```python
from build123d import *

# Parameters (mm, degrees)
SKETCH_1_R      = 1.6
EXTRUDE_1_DEPTH = 3
EXTRUDE_2_DEPTH = 10
SKETCH_3_R      = 1.6
EXTRUDE_3_DEPTH = 3


with BuildPart() as part:
    # 草图1 → 凸台-拉伸1 (new body)
    with BuildSketch(Plane(origin=(0, 0, 0), x_dir=(1, 0, 0), z_dir=(0, 1, 0))):
        with Locations(Location((0, 0, 0), (0, 0, 270))):
            Circle(SKETCH_1_R)
    extrude(amount=EXTRUDE_1_DEPTH)

    # 草图2 → 凸台-拉伸2 (add)
    with BuildSketch(Plane(origin=(0, 3, 0), x_dir=(1, 0, 0), z_dir=(0, 1, 0))):
        Polygon((2.757018897, -1.686460265), (2.839026881, 1.544418271), (0.082007983, 3.230878536), (-2.757018897, 1.686460265), (-2.839026881, -1.544418271), (-0.082007983, -3.230878536), align=None)
    extrude(amount=EXTRUDE_2_DEPTH)

    # 草图3 → 凸台-拉伸3 (add)
    with BuildSketch(Plane(origin=(0, 13, 0), x_dir=(1, 0, 0), z_dir=(0, 1, 0))):
        with Locations(Location((0, 0, 0), (0, 0, 270))):
            Circle(SKETCH_3_R)
    extrude(amount=EXTRUDE_3_DEPTH)


solid = part.part
```
Source: CAD feature listing. Evaluate the final solid. Frame: model axes, mm. A direction names the side the tool comes from. Give positions to 0.01 mm unless a question says otherwise; leave off trailing zeros. Loops run counter-clockwise (first coordinate to the right, second up) from the corner with the lowest first, then second, coordinate; pieces in that order, holes last. Notation, with made-up numbers: (46.25, -23.5) -> (66.25, -23.5) arc R9 cw to (66.25, -19.5) -> close; hole circle Ø11 at (52, -21.5). An arc over 180 degrees is marked (long way). Use a Markdown table: item, result. Add a question column.
(1) Access query for faces 1 (the face through (-0.97, 1.48, -1.27)), 2 (the face through (-1.48, 7.93, 2.376)), 3 (the face through (1.2, 13, 1.4)). Directions: +Z, -Z, +X, -X, +Y, -Y. A direction counts if a zero-diameter tool reaches every point of the face in a straight line with its end or side. Return the directions, or none.
(2) First-contact query: pin 1 Ø1 at (x, y) = (-2, 11) entering from +Z; pin 2 Ø1.5 at (x, y) = (1, 13) entering from +Z; pin 3 Ø1 at (y, z) = (12.5, 0) entering from -X. Flat tips, straight axial feed; report the tip coordinate or a pass-through.
(3) Section query A-A (y = 11.5). Output: boundary loops of the cut face in (x, z).
(4) Section query D-D (y = 1.5). Output: boundary loops of the cut face in (x, z).
(5) Section query B-B (z = -1.25). Output: boundary loops of the cut face in (x, y).
(6) Ray query, line 1 (Y direction, x = -0.2, z = 2.75); line 2 (X direction, y = 2.25, z = 0); line 3 (X direction, y = 8.5, z = -1.5). Return the intervals inside material, ascending.
(7) Section query C-C (x = -1.4). Output: boundary loops of the cut face in (y, z), then the cut area to 3 significant figures.
Checked values:
| question | item | result |
|---|---|---|
| 1 | face 1 | -Y |
| 1 | face 2 | +Z, -X, +Y, -Y |
| 1 | face 3 | +Y |
| 2 | pin 1 | z = 2.36 |
| 2 | pin 2 | z = 3.05 |
| 2 | pin 3 | x = -2.81 |
| 3 | outline | (-2.84, 1.54) -> (-2.76, -1.69) -> (0.08, -3.23) -> (2.84, -1.54) -> (2.76, 1.69) -> (-0.08, 3.23) -> close |
| 4 | outline | circle Ø3.2 at (0, 0) |
| 5 | outline | (-2.77, 3) -> (-1, 3) -> (-1, 0) -> (1, 0) -> (1, 3) -> (2.83, 3) -> (2.83, 13) -> (1, 13) -> (1, 16) -> (-1, 16) -> (-1, 13) -> (-2.77, 13) -> close |
| 6 | line 1 | 3 to 13 |
| 6 | line 2 | -1.6 to 1.6 |
| 6 | line 3 | -2.76 to 2.84 |
| 7 | outline | (0, -0.77) -> (3, -0.77) -> (3, -2.42) -> (13, -2.42) -> (13, -0.77) -> (16, -0.77) -> (16, 0.77) -> (13, 0.77) -> (13, 2.42) -> (3, 2.42) -> (3, 0.77) -> (0, 0.77) -> close |
| 7 | area | 57.8 mm^2 |
